Work out the finished part from the listing and answer in its coordinate system (mm). Face numbers are marked on the shaded views. A direction names the side the tool comes from. Coordinates: 2 decimals unless noted, no trailing zeros. Write each loop counter-clockwise with the first axis right and the second up, starting at its lowest first coordinate (ties: lowest second). Pieces come first, ordered by that corner, then holes. Notation, with made-up numbers: (59, 89) - (93, 89) arc R16 cw to (93, 113) - close; hole circle Ø4 at (73, 31.25). An arc over 180 degrees is marked (long way). Use one line per item in the form item = value. Start each with the question number.
Item 1: Determine the mould class of the marked faces 4, 5, 6 and 7 for opening direction X: released by +X, released by -X, zero draft, split by the parting line, or undercut.
Item 2: Given pin 1 (12 mm diameter, centred on x = -39, z = 48.5, fed in from -Y); pin 2 (24 mm diameter, centred on x = 0, y = -150, fed in from -Z); pin 3 (15 mm diameter, centred on x = -12, z = 41.5, fed in from +Y); pin 4 (6 mm diameter, centred on x = 25, y = -120, fed in from +Z), each flat-ended and moving along its own axis, determine where each tip first touches the part or whether it passes through.
Item 3: A cutting plane is placed at D-D (y = 120). Write down the section's boundary in (x, z), then the cut area to 3 significant figures.
Item 4: A cutting plane is placed at C-C (z = 68). Write down the section's boundary in (x, y), then the cut area to 3 significant figures.
Item 5: A cutting plane is placed at B-B (z = 6). Write down the section's boundary in (x, y).
Item 6: For the marked faces 1, 2 and 3, determine the directions among +Z, -Z, +X, -X, +Y, -Y from which every point of the face is accessible in a straight line to the end or side of a thin tool.
Item 7: A cutting plane is placed at A-A (x = 0). Give the number of separate pieces and of enclosed holes in the cut face, then the cut area to 3 significant figures.
Item 8: Consider probe 1 along X at (y, z) = (-120, 76); probe 2 along Y at (x, z) = (0, 7); probe 3 along Y at (x, z) = (25, 74). Determine where each line is inside the solid, lowest interval first.
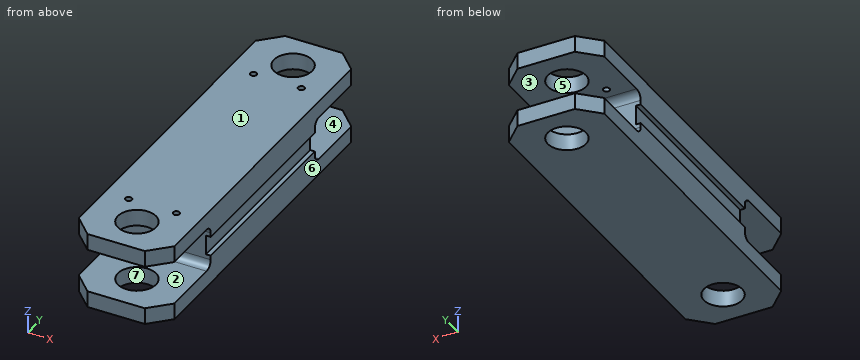
from build123d import *

# Parameters (mm, degrees)
SKETCH_1_W              = 100
SKETCH_1_H              = 380
EXTRUDE_1_DEPTH         = 80
CUT_EXTRUDE_1_REACH     = 231.129
SKETCH_2_W              = 45.5
SKETCH_2_H              = 90
SKETCH_3_W              = 20.5
SKETCH_3_H              = 290
CUT_EXTRUDE_2_DEPTH     = 5
SKETCH_4_R              = 20
CUT_EXTRUDE_3_DEPTH     = 213.132034356
HOLE_WIZARD_M8_1_REACH  = 214.132
HOLE_WIZARD_M8_1_BORE_R = 3.4
FILLET_1_R              = 8
CHAMFER_1_SIZE          = 20


with BuildPart() as part:
    # Sketch 1 → Extrude 1 (new body)
    with BuildSketch(Plane.XY):
        Rectangle(SKETCH_1_W, SKETCH_1_H)
    extrude(amount=EXTRUDE_1_DEPTH)

    # Sketch 2 → Cut-Extrude 1 (cut, up to next)
    with BuildSketch(Plane(origin=(50, 0, 0), x_dir=(0, 0, -1), z_dir=(1, 0, 0)), mode=Mode.PRIVATE) as cut_extrude_1_sk1:
        with Locations((-40, 145)):
            Rectangle(SKETCH_2_W, SKETCH_2_H)
    cut_extrude_1_tool1 = extrude(cut_extrude_1_sk1.sketch, amount=-CUT_EXTRUDE_1_REACH, mode=Mode.PRIVATE) & part.part
    cut_extrude_1 = cut_extrude_1_tool1.solids().sort_by_distance((50, 145, 40))[0]
    add(cut_extrude_1, mode=Mode.SUBTRACT)

    # Sketch 3 → Cut-Extrude 2 (cut)
    with BuildSketch(Plane(origin=(50, 0, 0), x_dir=(0, 0, -1), z_dir=(1, 0, 0))):
        with Locations((-40, -45)):
            Rectangle(SKETCH_3_W, SKETCH_3_H)
    cut_extrude_2 = extrude(amount=-CUT_EXTRUDE_2_DEPTH, mode=Mode.SUBTRACT)

    # Mirror 1: Cut-Extrude 1 across plane
    add(cut_extrude_1.mirror(Plane.ZX), mode=Mode.SUBTRACT)

    # Mirror 2: Cut-Extrude 2 across plane
    add(cut_extrude_2.mirror(Plane(origin=(0, 0, 0), x_dir=(0, 0, 1), z_dir=(1, 0, 0))), mode=Mode.SUBTRACT)

    # Sketch 4 → Cut-Extrude 3 (cut, through all)
    with BuildSketch(Plane.XY.offset(80)):
        with Locations((0, 150)):
            Circle(SKETCH_4_R)
    cut_extrude_3 = extrude(amount=-CUT_EXTRUDE_3_DEPTH, mode=Mode.SUBTRACT)

    # Mirror 3: Cut-Extrude 3 across plane
    add(cut_extrude_3.mirror(Plane.ZX), mode=Mode.SUBTRACT)

    # Hole Wizard M8 _1 bore → Hole Wizard M8 _1 (cut, up to next)
    with BuildSketch(Plane.XY.offset(80), mode=Mode.PRIVATE) as hole_wizard_m8_1_sk1:
        with Locations((-25, 120)):
            Circle(HOLE_WIZARD_M8_1_BORE_R)
    hole_wizard_m8_1_tool1 = extrude(hole_wizard_m8_1_sk1.sketch, amount=-HOLE_WIZARD_M8_1_REACH, mode=Mode.PRIVATE) & part.part
    # Hole Wizard M8 _1 bore → Hole Wizard M8 _1 (cut, up to next)
    with BuildSketch(Plane.XY.offset(80), mode=Mode.PRIVATE) as hole_wizard_m8_1_sk2:
        with Locations((25, 120)):
            Circle(HOLE_WIZARD_M8_1_BORE_R)
    hole_wizard_m8_1_tool2 = extrude(hole_wizard_m8_1_sk2.sketch, amount=-HOLE_WIZARD_M8_1_REACH, mode=Mode.PRIVATE) & part.part
    hole_wizard_m8_1_1 = hole_wizard_m8_1_tool1.solids().sort_by_distance((-25, 120, 80))[0]
    add(hole_wizard_m8_1_1, mode=Mode.SUBTRACT)
    hole_wizard_m8_1_2 = hole_wizard_m8_1_tool2.solids().sort_by_distance((25, 120, 80))[0]
    add(hole_wizard_m8_1_2, mode=Mode.SUBTRACT)
    hole_wizard_m8_1 = hole_wizard_m8_1_1 + hole_wizard_m8_1_2  # Hole Wizard M8 _1 as one shape, for the pattern or mirror that repeats it

    # Mirror 4: Hole Wizard M8 _1 across plane
    add(hole_wizard_m8_1.mirror(Plane.ZX), mode=Mode.SUBTRACT)

    # Fillet 1
    fillet_1_edges = [part.edges().sort_by_distance(p)[0] for p in [
        (0, 100, 17.25),
        (0, 100, 62.75),
        (0, -100, 62.75),
        (0, -100, 17.25),
    ]]
    fillet(fillet_1_edges, radius=FILLET_1_R)

    # Chamfer 1
    chamfer_1_edges = [part.edges().sort_by_distance(p)[0] for p in [
        (-50, 190, 8.625),
        (50, 190, 8.625),
        (50, -190, 8.625),
        (-50, -190, 8.625),
        (-50, 190, 71.375),
        (50, 190, 71.375),
        (50, -190, 71.375),
        (-50, -190, 71.375),
    ]]
    chamfer(chamfer_1_edges, length=CHAMFER_1_SIZE)


solid = part.part
Answer:
q1.face_4 = zero draft
q1.face_5 = undercut
q1.face_6 = released by +X
q1.face_7 = undercut
q2.pin_1 = -100
q2.pin_2 = through
q2.pin_3 = 100
q2.pin_4 = 17.25
q3.outline = (-50, 0) - (50, 0) - (50, 17.25) - (-50, 17.25) - close; (-50, 62.75) - (-28.4, 62.75) - (-28.4, 80) - (-50, 80) - close; (-21.6, 62.75) - (21.6, 62.75) - (21.6, 80) - (-21.6, 80) - close; (28.4, 62.75) - (50, 62.75) - (50, 80) - (28.4, 80) - close
q3.area = 3,220 mm²
q4.outline = (-50, -170) - (-30, -190) - (30, -190) - (50, -170) - (50, 170) - (30, 190) - (-30, 190) - (-50, 170) - close; hole circle Ø6.8 at (-25, -120); hole circle Ø6.8 at (-25, 120); hole circle Ø40 at (0, -150); hole circle Ø40 at (0, 150); hole circle Ø6.8 at (25, -120); hole circle Ø6.8 at (25, 120)
q4.area = 34,500 mm²
q5.outline = (-50, -170) - (-30, -190) - (30, -190) - (50, -170) - (50, 170) - (30, 190) - (-30, 190) - (-50, 170) - close; hole circle Ø40 at (0, -150); hole circle Ø40 at (0, 150)
q6.face_1 = +Z, +X, -X, +Y, -Y
q6.face_2 = +X, -X, -Y
q6.face_3 = +X, -X, +Y
q7.separate_pieces = 5
q7.enclosed_holes = 0
q7.area = 19,500 mm²
q8.probe_1 = -50 to -28.4, -21.6 to 21.6, 28.4 to 50
q8.probe_2 = -190 to -170, -130 to 130, 170 to 190
q8.probe_3 = -190 to -123.4, -116.6 to 116.6, 123.4 to 190
